Source: CAD feature listing. Evaluate the final solid. Frame: model axes, mm. Give positions to 0.01 mm unless a question says otherwise; leave off trailing zeros. Order: outer loops, then holes, each group sorted by start corner. A loop starts at its lowest first (then second) coordinate and runs counter-clockwise, first axis right, second up. Notation, with made-up numbers: (-7, 57.5) -> (18, 57.5) arc R15 ccw to (18, 81.5) -> close; hole circle Ø11 at (35, 77). An arc over 180 degrees is marked (long way). Answer in a Markdown table with one row per item.
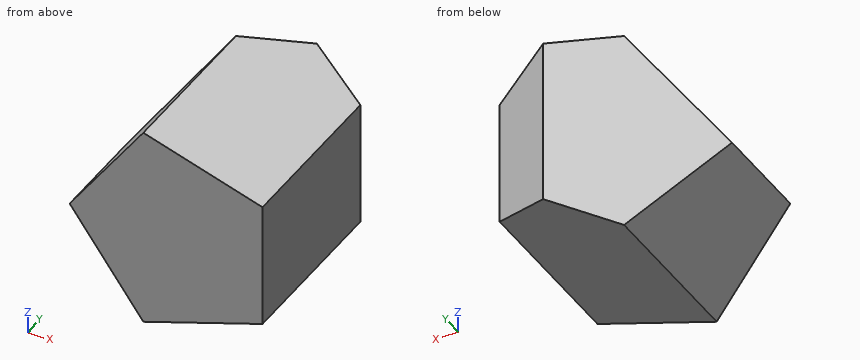
Autodesk Inventor part; units mm, degrees
ref_plane "YZ Plane" through (0, 0, 0) normal (1, 0, 0) x (0, 1, 0)
ref_plane "XZ Plane" through (0, 0, 0) normal (0, 1, 0) x (-1, 0, 0)
ref_plane "XY Plane" through (0, 0, 0) normal (0, 0, 1) x (1, 0, 0)
sketch "Эскиз3" plane through (0, 0, 0) normal (1, 0, 0) x (0, 1, 0)
  line L0 (50, 7.7254) -> (50, -20.2254)
  line L1 (50, -6.25) -> (41.9313, -20.2254)
  line L2 (50, -6.25) -> (23.7781, 25)
  line L3 (50, 25) -> (50, 7.7254)
  line L4 (0, -20.2254) -> (50, -20.2254)
  line L5 (0, 25) -> (50, 25)
  line L6 (23.7781, 25) -> (25, -20.2254)
  point P0 (0, 0)
  dimension "d4" = 140
  dimension "d5" = 150
extrude "Выдавливание2" [suppressed]
sketch "Эскиз4" plane through (0, 0, 0) normal (1, 0, 0) x (0, 1, 0)
  line L0 (50, -20.2254) -> (50, -6.25)
  line L1 (50, -6.25) -> (41.9313, -20.2254)
  line L2 (0, -20.2254) -> (50, -20.2254)
  line L3 (50, -6.25) -> (66.1374, -6.25) construction
  point P0 (0, 0)
  dimension "d8" = 120
extrude "Выдавливание3" [suppressed]
sketch "Эскиз5" plane through (0, 0, 0) normal (0, 1, 0) x (-1, 0, 0)
  circle A0 centre (0, 0) radius 25
  line L0 (25, 0) -> (7.7254, -23.7764)
  line L1 (7.7254, -23.7764) -> (-20.2254, -14.6946)
  line L2 (-20.2254, -14.6946) -> (-20.2254, 14.6946)
  line L3 (-20.2254, 14.6946) -> (7.7254, 23.7764)
  line L4 (7.7254, 23.7764) -> (25, 0)
  dimension "d11" = 50
extrude "Выдавливание4" add sketch "Эскиз5" along normal blind 50 contours L0 L1 L2 L3 L4
sketch "Эскиз6" plane through (0, 50, 0) normal (0, 1, 0) x (1, 0, 0)
  line L0 (-7.7254, -23.7764) -> (20.2254, -14.6946)
  line L1 (5.2254, -19.5684) -> (5.2254, 19.5684)
  line L2 (20.2254, 14.6946) -> (-7.7254, 23.7764)
  line L3 (20.2254, -14.6946) -> (20.2254, 14.6946)
  point P0 (0, 0)
  dimension "d14" = 15
sketch "Эскиз7" plane through (0, 0, 0) normal (0, 0, 1) x (1, 0, 0)
  line L0 (-7.7254, 50) -> (20.2254, 50)
  line L1 (20.2254, 50) -> (5.2254, 50)
  line L2 (5.2254, 50) -> (20.2254, 41.3397)
  line L3 (20.2254, 0) -> (20.2254, 50)
  line L4 (5.2254, 50) -> (22.5459, 50) construction
  line L5 (20.2254, 41.3397) -> (20.2254, 50)
  point P0 (0, 0)
  dimension "d15" = 15
  dimension "d16" = 30
extrude "Выдавливание5" cut sketch "Эскиз7" along normal mid plane 50
sketch "Эскиз8" plane through (0, 0, 0) normal (0, 0, 1) x (1, 0, 0)
  line L0 (-25, 50) -> (-7.7254, 50)
  line L1 (-25, 50) -> (5.2254, 50)
  line L2 (5.2254, 50) -> (-25, 24.6379)
  line L3 (-25, 0) -> (-25, 50)
  line L4 (-25, 24.6379) -> (-25, 50)
  point P0 (0, 0)
  dimension "d19" = 40
extrude "Выдавливание6" cut sketch "Эскиз8" along normal mid plane 50
properties part number "Призма"
(1) Ray query, probe 1 along Y at (x, z) = (11, 8.5); probe 2 along Y at (x, z) = (5, -5); probe 3 along X at (y, z) = (9, -14.5). Return the intervals inside material, ascending.
A:
| item | result |
|---|---|
| probe 1 | y = 0 to 46.67 |
| probe 2 | y = 0 to 49.81 |
| probe 3 | x = -14.47 to 20.23 |
(2) Section query C-C (z = -3.5). Return the cut outline in (x, y), plus the area to 3 significant figures.
A:
| item | result |
|---|---|
| outline | (-22.46, 0) -> (20.23, 0) -> (20.23, 41.34) -> (5.23, 50) -> (-22.46, 26.77) -> close |
| area | 1,750 mm^2 |
(3) Section query D-D (y = 46.5). Return the cut outline in (x, z).
A:
| item | result |
|---|---|
| outline | (1.05, -20.92) -> (11.29, -17.6) -> (11.29, 17.6) -> (1.05, 20.92) -> close |
(4) Section query B-B (x = -19.5). Return the cut outline in (y, z), plus the area to 3 significant figures.
A:
| item | result |
|---|---|
| outline | (0, -7.57) -> (29.25, -7.57) -> (29.25, 7.57) -> (0, 7.57) -> close |
| area | 443 mm^2 |
(5) First-contact query: pin 1 Ø12 at (x, y) = (1.5, 42.5) entering from -Z; pin 2 Ø8 at (x, z) = (8, -4.5) entering from -Y; pin 3 Ø10 at (x, z) = (4.5, -10) entering from +Y; pin 4 Ø6 at (x, y) = (9, 27) entering from -Z. Flat tips, straight axial feed; report the tip coordinate or a pass-through.
A:
| item | result |
|---|---|
| pin 1 | stops at z = -22.72 |
| pin 2 | stops at y = 0 |
| pin 3 | stops at y = 50 |
| pin 4 | stops at z = -19.32 |
(6) Section query A-A (z = 16). Return the cut outline in (x, y).
A:
| item | result |
|---|---|
| outline | (-13.38, 0) -> (16.21, 0) -> (16.21, 43.66) -> (5.23, 50) -> (-13.38, 34.39) -> close |
